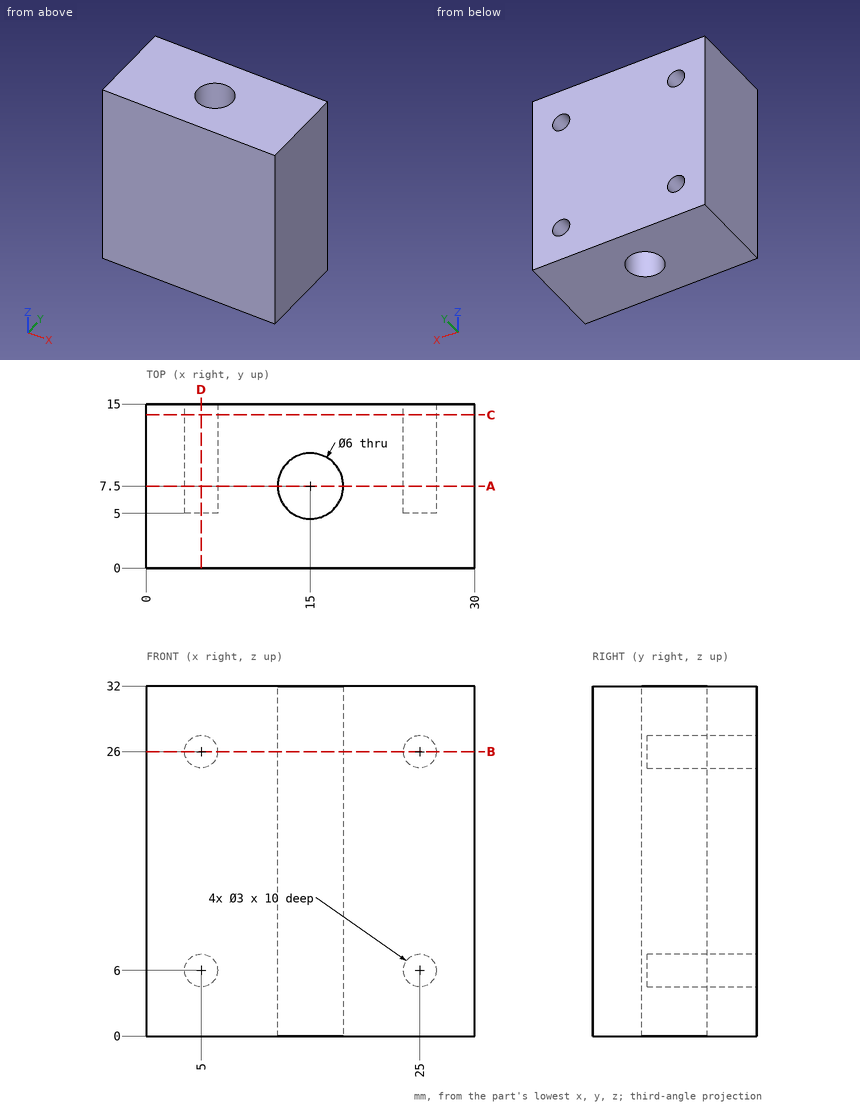
Verification items for this drawing (mm, ordinates from the low corner). Give positions to 0.01 mm unless a question says otherwise; leave off trailing zeros. Write each loop counter-clockwise with the first axis right and the second up, starting at its lowest first coordinate (ties: lowest second). Pieces come first, ordered by that corner, then holes.
1) Thickness scan on line 1 (Z direction, x = 5, y = 11.5); line 2 (X direction, y = 12, z = 6); line 3 (X direction, y = 8.25, z = 26). Record the ranges inside material, lowest first.
Values follow:
line 1: z = 0 to 4.5, 7.5 to 24.5, 27.5 to 32
line 2: x = 0 to 3.5, 6.5 to 23.5, 26.5 to 30
line 3: x = 0 to 3.5, 6.5 to 12.1, 17.9 to 23.5, 26.5 to 30
2) Cross-section at D-D (x = 5). Record the boundary of the cut face in (y, z), plus the area to 3 significant figures.
Values follow:
outline: (0, 0) - (15, 0) - (15, 4.5) - (5, 4.5) - (5, 7.5) - (15, 7.5) - (15, 24.5) - (5, 24.5) - (5, 27.5) - (15, 27.5) - (15, 32) - (0, 32) - close
area: 420 mm2
3) Cross-section at C-C (y = 14). Record the boundary of the cut face in (x, z), plus the area to 3 significant figures.
Values follow:
outline: (0, 0) - (30, 0) - (30, 32) - (0, 32) - close; hole circle Ø3 at (5, 6); hole circle Ø3 at (5, 26); hole circle Ø3 at (25, 6); hole circle Ø3 at (25, 26)
area: 932 mm2
4) Cross-section at A-A (y = 7.5). Record the boundary of the cut face in (x, z).
Values follow:
outline: (0, 0) - (12, 0) - (12, 32) - (0, 32) - close; (18, 0) - (30, 0) - (30, 32) - (18, 32) - close; hole circle Ø3 at (5, 6); hole circle Ø3 at (5, 26); hole circle Ø3 at (25, 6); hole circle Ø3 at (25, 26)
5) Cross-section at B-B (z = 26). Record the boundary of the cut face in (x, y).
Values follow:
outline: (0, 0) - (30, 0) - (30, 15) - (26.5, 15) - (26.5, 5) - (23.5, 5) - (23.5, 15) - (6.5, 15) - (6.5, 5) - (3.5, 5) - (3.5, 15) - (0, 15) - close; hole circle Ø6 at (15, 7.5)
6) Go/stop test with flat-tipped pins: pin 1 Ø2.5 at (x, z) = (25.5, 5.5) entering from +Y; pin 2 Ø2.5 at (x, z) = (25, 6) entering from +Y. Record where each tip stops, or that it passes through.
Values follow:
pin 1: stops at y = 15
pin 2: stops at y = 5
